Study the drawing (mm; zero at the part's minimum x, y, z) and answer. A direction names the side the tool comes from. Coordinates: 2 decimals unless noted, no trailing zeros. Order: outer loops, then holes, each group sorted by start corner. A loop starts at its lowest first (then second) coordinate and runs counter-clockwise, first axis right, second up.
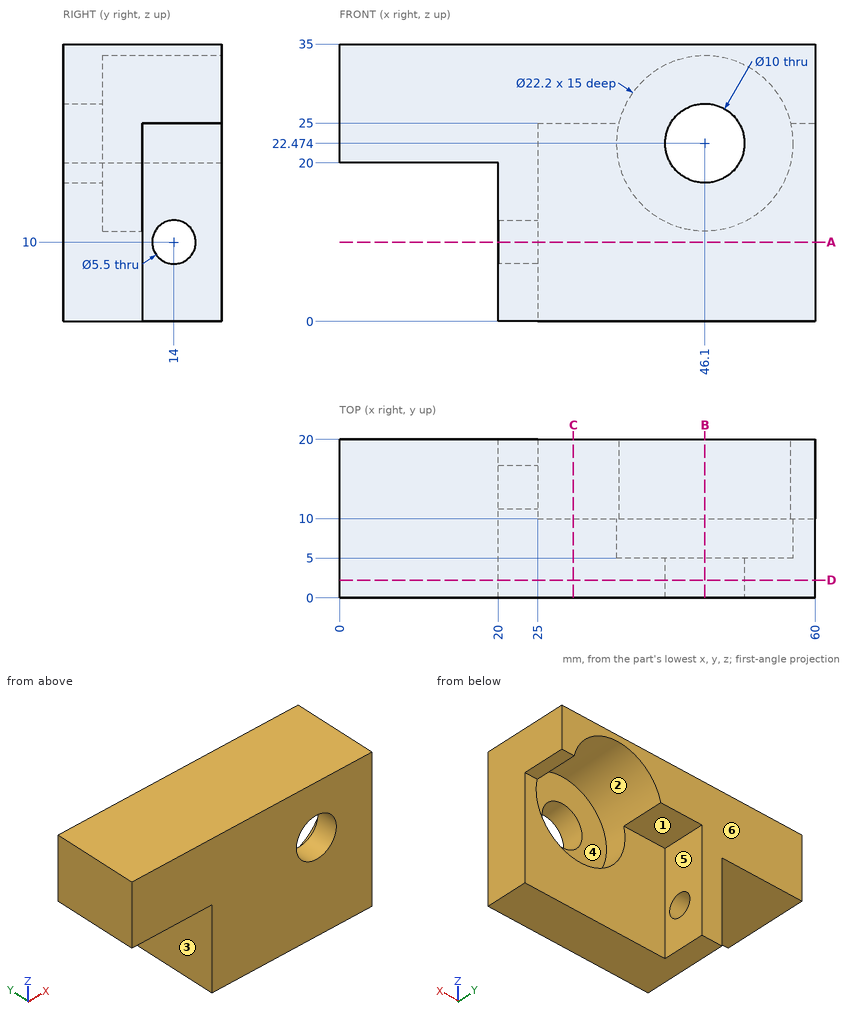
1) Which of the six approach directions +Z, -Z, +X, -X, +Y, -Y give full straight-line access (tool end or side, diameter ignored) to the marked faces 1, 2 and 3?
A:
face 1: -Z, +X, +Y
face 2: +Y
face 3: -Z, -X, +Y, -Y
2) Determine the mould class of the marked faces 4, 5 and 6 for opening direction X: pulls with the +X half, pulls with the -X half, needs draft (parallel to the pull), parting line crosses it, or undercut.
A:
face 4: undercut
face 5: pulls with the +X half
face 6: needs draft
3) Flat-ended cylindrical pins translate along their axes: pin 1 Ø2 at (y, z) = (15.5, 23) entering from +X; pin 2 Ø0.9 at (x, y) = (59, 16) entering from -Z; pin 3 Ø7.5 at (x, z) = (37.5, 10.5) entering from +Y. Find the tip coordinate at first contact, or state that the pin passes through.
A:
pin 1: stops at x = 25
pin 2: stops at z = 25
pin 3: stops at y = 10
4) A cutting plane is placed at B-B, the plane x = 46.1. Determine the outline of the cut face in (y, z), and give its area (3 significant figures).
A:
outline: (0, 0) - (10, 0) - (10, 11.37) - (5, 11.37) - (5, 17.47) - (0, 17.47) - close; (0, 27.47) - (5, 27.47) - (5, 33.57) - (20, 33.57) - (20, 35) - (0, 35) - close
area: 203 mm2
5) A cutting plane is placed at A-A, the plane z = 10. Determine the outline of the cut face in (x, y).
A:
outline: (20, 0) - (60, 0) - (60, 10) - (25, 10) - (25, 11.25) - (20, 11.25) - close; (20, 16.75) - (25, 16.75) - (25, 20) - (20, 20) - close
6) A cutting plane is placed at D-D, the plane y = 2.25. Determine the outline of the cut face in (x, z).
A:
outline: (0, 20) - (20, 20) - (20, 0) - (60, 0) - (60, 35) - (0, 35) - close; hole circle Ø10 at (46.1, 22.47)
7) Straight lines are drawn through the part: line 1 (Z direction, x = 46.1, y = 2.2); line 2 (X direction, y = 9, z = 23); line 3 (Y direction, x = 53, z = 23). For each, find the intervals that lie inside material, in ascending order.
A:
line 1: z = 0 to 17.47, 27.47 to 35
line 2: x = 0 to 35.01, 57.19 to 60
line 3: y = 0 to 5
8) A cutting plane is placed at C-C, the plane x = 29.5. Determine the outline of the cut face in (y, z), and give its area (3 significant figures).
A:
outline: (0, 0) - (10, 0) - (10, 25) - (20, 25) - (20, 35) - (0, 35) - close
area: 450 mm2
